Autodesk Inventor part; units mm, degrees
ref_plane "YZ Plane" through (0, 0, 0) normal (1, 0, 0) x (0, 1, 0)
ref_plane "XZ Plane" through (0, 0, 0) normal (0, 1, 0) x (-1, 0, 0)
ref_plane "XY Plane" through (0, 0, 0) normal (0, 0, 1) x (1, 0, 0)
sketch "スケッチ3" plane through (0, 0, 0) normal (0, 1, 0) x (-1, 0, 0)
  circle A0 centre (55.3, 11.85) radius 2.1
  circle A1 centre (31.1, 14.7) radius 2.1
  circle A2 centre (6.9, 11.85) radius 2.1
  line L0 (62.1, 5.5) -> (0.1, 5.5)
  line L1 (2.1, 20) -> (60.1, 20)
  line L2 (-0.9, 6.5) -> (-0.9, 17)
  line L3 (63.1, 17) -> (63.1, 6.5)
  line L4 (49.3, -20) -> (41.3, -20)
  line L5 (21.3, -20) -> (13.3, -20)
  line L6 (63.1, 17) -> (60.1, 20)
  line L7 (2.1, 20) -> (-0.9, 17)
  line L8 (50.3, -19) -> (50.3, 5.5)
  line L9 (40.3, -19) -> (40.3, 5.5)
  line L10 (22.3, -19) -> (22.3, 5.5)
  line L11 (12.3, -19) -> (12.3, 5.5)
  line L12 (62.1, 5.5) -> (63.1, 6.5)
  line L13 (0.1, 5.5) -> (-0.9, 6.5)
  line L14 (12.3, -19) -> (13.3, -20)
  line L15 (22.3, -19) -> (21.3, -20)
  line L16 (40.3, -19) -> (41.3, -20)
  line L17 (50.3, -19) -> (49.3, -20)
  point P0 (0, 0)
  point P1 (-0.9, 20)
  point P2 (-0.9, 5.5)
  point P3 (63.1, 5.5)
  point P4 (50.3, -20)
  point P5 (40.3, -20)
  point P6 (22.3, -20)
  point P7 (12.3, -20)
  point P8 (61.6, 18.5)
  dimension "d2" = 3
  dimension "d3" = 3
  dimension "d4" = 4.2
  dimension "d5" = 4.2
  dimension "d6" = 4.2
  dimension "d7" = 10
  dimension "d8" = 10
  dimension "d11" = 1
  dimension "d12" = 1
  dimension "d13" = 1
  dimension "d14" = 1
  dimension "d16" = 1
  dimension "d17" = 1
  dimension "d18" = 1
  dimension "d19" = 1
  dimension "d20" = 1
  dimension "d21" = 1
  dimension "d22" = 1
extrude "押し出し1" add sketch "スケッチ3" along normal blind 3
sketch "スケッチ4" plane through (0, 0, 0) normal (0, -1, 0) x (1, 0, 0)
  line L0 (-40.3, 5.5) -> (-22.3, 5.5)
  line L1 (-22.3, 5.5) -> (-22.3, -6.5)
  line L2 (-22.3, -6.5) -> (-40.3, -6.5)
  line L3 (-40.3, -6.5) -> (-40.3, 5.5)
  line L4 (-22.3, -19) -> (-22.3, 5.5)
  point P0 (0, 0)
  dimension "d23" = 12
extrude "押し出し2" add sketch "スケッチ4" against normal blind 3
sketch "スケッチ5" plane through (0, 0, 0) normal (0, -1, 0) x (1, 0, 0)
  line L0 (-0.1, 5.5) -> (-12.3, 5.5)
  line L1 (-12.3, 5.5) -> (-12.3, -6.7)
  line L2 (-12.3, -6.7) -> (-0.1, 5.5)
  line L3 (0.9, 6.5) -> (-0.1, 5.5)
  line L4 (-50.3, -6.3) -> (-50.3, 5.5)
  line L5 (-50.3, 5.5) -> (-62.1, 5.5)
  line L6 (-62.1, 5.5) -> (-50.3, -6.3)
  line L7 (-62.1, 5.5) -> (-63.1, 6.5)
  point P0 (0, 0)
extrude "押し出し3" add sketch "スケッチ5" against normal blind 3
fillet "フィレット2" radius 8 2 edges at (-22.3, 1.5, -6.5) (-40.3, 1.5, -6.5)
fillet "フィレット2" radius 16 2 edges at (-12.3, 1.5, -6.7) (-50.3, 1.5, -6.3)
equation "\"d7\" = d8"
equation "\"d15\" = d11"
properties part number "stopperver2_2"
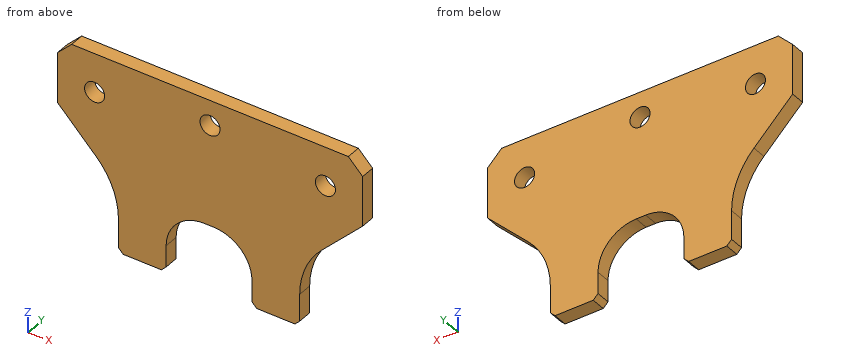
Source: CAD feature listing. Evaluate the final solid. Frame: model axes, mm. Coordinates: 2 decimals unless noted, no trailing zeros. Write each loop counter-clockwise with the first axis right and the second up, starting at its lowest first coordinate (ties: lowest second). Pieces come first, ordered by that corner, then holes. Notation, with made-up numbers: M 64,-2.5 L 121,-2.5 A4 ccw 121,4.5 Z; hole C 37,63 d10. An arc over 180 degrees is marked long. Use a Markdown table: item, result.
1) Section B-B, the plane z = 14.7. Output: boundary loops of the cut face in (x, y), then the cut area to 3 significant figures.
Conclusion:
| item | result |
|---|---|
| outline | M -63.1,0 L -33.2,0 L -33.2,3 L -63.1,3 Z; M -29,0 L 0.9,0 L 0.9,3 L -29,3 Z |
| area | 179 mm^2 |
2) Section A-A, the plane x = -6.9. Output: boundary loops of the cut face in (y, z), then the cut area to 3 significant figures.
Conclusion:
| item | result |
|---|---|
| outline | M 0,-1.3 L 3,-1.3 L 3,9.75 L 0,9.75 Z; M 0,13.95 L 3,13.95 L 3,20 L 0,20 Z |
| area | 51.3 mm^2 |
3) First-contact query: pin 1 Ø1 at (y, z) = (1, -13.5) entering from +X; pin 2 Ø0.9 at (y, z) = (1.5, -16.5) entering from -X; pin 3 Ø1 at (x, y) = (-31.5, 1) entering from -Z; pin 4 Ø3.5 at (x, z) = (-6.9, 11.85) entering from -Y. Flat tips, straight axial feed; report the tip coordinate or a pass-through.
Conclusion:
| item | result |
|---|---|
| pin 1 | stops at x = -12.3 |
| pin 2 | stops at x = -50.3 |
| pin 3 | stops at z = -6.5 |
| pin 4 | passes through |
4) Section C-C, the plane y = 0.8. Output: boundary loops of the cut face in (x, z), then the cut area to 3 significant figures.
Conclusion:
| item | result |
|---|---|
| outline | M -63.1,6.5 L -54.99,-1.61 A16 cw -50.3,-12.93 L -50.3,-19 L -49.3,-20 L -41.3,-20 L -40.3,-19 L -40.3,-14.5 A8 cw -32.3,-6.5 L -30.3,-6.5 A8 cw -22.3,-14.5 L -22.3,-19 L -21.3,-20 L -13.3,-20 L -12.3,-19 L -12.3,-13.33 A16 cw -7.61,-2.01 L 0.9,6.5 L 0.9,17 L -2.1,20 L -60.1,20 L -63.1,17 Z; hole C -55.3,11.85 d4.2; hole C -31.1,14.7 d4.2; hole C -6.9,11.85 d4.2 |
| area | 1,780 mm^2 |
5) Section D-D, the plane z = 5.5. Output: boundary loops of the cut face in (x, y).
Conclusion:
| item | result |
|---|---|
| outline | M -62.1,0 L -0.1,0 L -0.1,3 L -62.1,3 Z |
6) Ray query, L1, parallel to X at y = 0.65, z = -15.5; L2, parallel to Z at x = -31.1, y = 1.7; L3, parallel to X at y = 2.5, z = -12. Return the intervals inside material, ascending.
Conclusion:
| item | result |
|---|---|
| L1 | x = -50.3 to -40.3, -22.3 to -12.3 |
| L2 | z = -6.5 to 12.6, 16.8 to 20 |
| L3 | x = -50.33 to -39.9, -22.7 to -12.24 |
